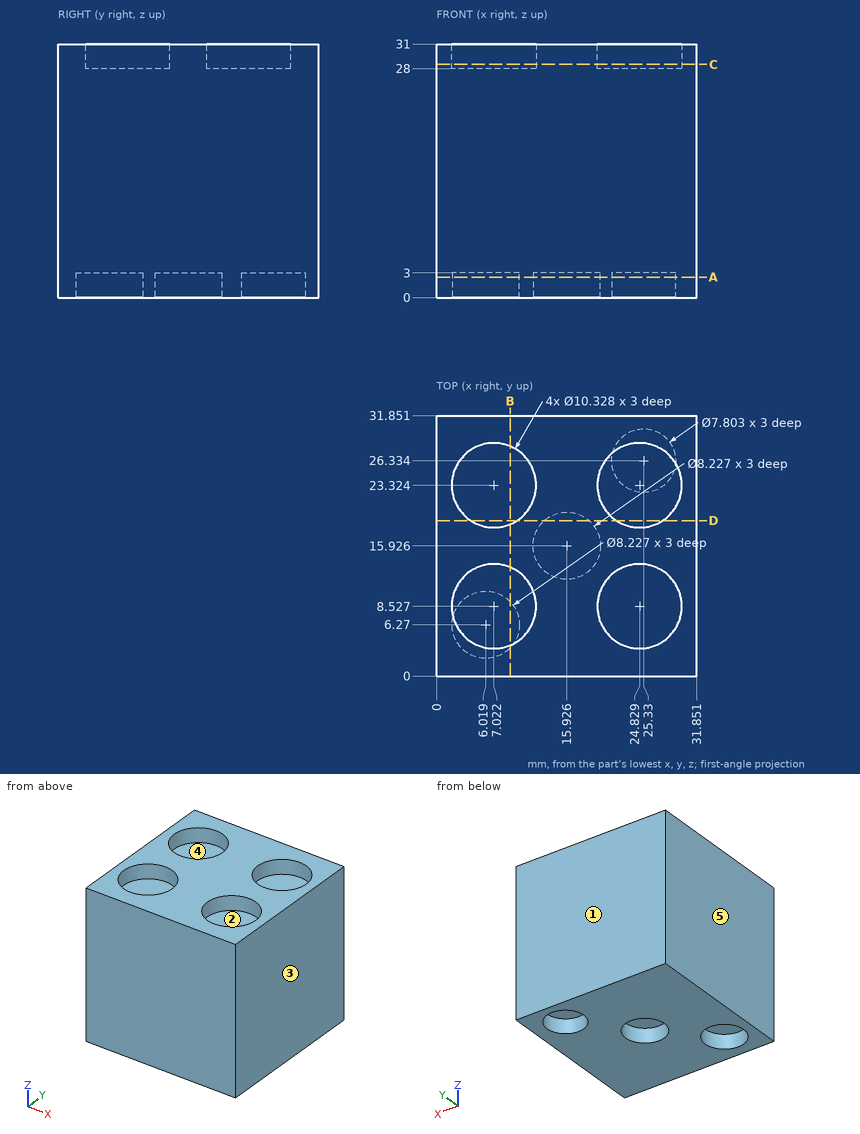
Verification items for this drawing (mm, ordinates from the low corner). A direction names the side the tool comes from. Round coordinates to 2 decimals unless told otherwise and drop trailing zeros. Order: outer loops, then holes, each group sorted by start corner. A loop starts at its lowest first (then second) coordinate and runs counter-clockwise, first axis right, second up. Notation, with made-up numbers: (2, 62.25) -> (50, 62.25) arc R16 ccw to (50, 88.25) -> close; hole circle Ø10 at (13, -34). An arc over 180 degrees is marked (long way). Use one line per item in the form item = value.
1. Mould release check, pull along Y, two halves, no side actions. Record for the marked faces 1, 2 and 3: pulls with the +Y half, pulls with the -Y half, needs draft (parallel to the pull), parting line crosses it, or undercut.
Working result:
face_1 = pulls with the +Y half
face_2 = undercut
face_3 = needs draft
2. Cross-section at C-C, the plane z = 28.5. Enter the section's corners in (x, y) (1 decimal).
Working result:
outline = (0, 0) -> (31.9, 0) -> (31.9, 31.9) -> (0, 31.9) -> close; hole circle Ø10.3 at (7, 8.5); hole circle Ø10.3 at (7, 23.3); hole circle Ø10.3 at (24.8, 8.5); hole circle Ø10.3 at (24.8, 23.3)
3. Set-up check for the marked faces 4 and 5: record each of +Z, -Z, +X, -X, +Y, -Y from which the full face is reachable in a straight line by a thin tool's end or side.
Working result:
face_4 = +Z
face_5 = +Z, -Z, -X, +Y, -Y
4. Cross-section at D-D, the plane y = 19. Enter the section's corners in (x, z) (1 decimal).
Working result:
outline = (0, 0) -> (13.2, 0) -> (13.2, 3) -> (18.7, 3) -> (18.7, 0) -> (31.9, 0) -> (31.9, 31) -> (27.7, 31) -> (27.7, 28) -> (22, 28) -> (22, 31) -> (9.8, 31) -> (9.8, 28) -> (4.2, 28) -> (4.2, 31) -> (0, 31) -> close
5. Cross-section at B-B, the plane x = 9. Enter the section's corners in (y, z) (1 decimal), plus the area to 3 significant figures.
Working result:
outline = (0, 0) -> (3.4, 0) -> (3.4, 3) -> (9.1, 3) -> (9.1, 0) -> (31.9, 0) -> (31.9, 31) -> (28.1, 31) -> (28.1, 28) -> (18.6, 28) -> (18.6, 31) -> (13.3, 31) -> (13.3, 28) -> (3.8, 28) -> (3.8, 31) -> (0, 31) -> close
area = 913 mm^2
6. Scan lines: line 1 along Z through (x, y) = (28.5, 27); line 2 along Z through (x, y) = (29, 23). Record each from-to range of solid material in increasing order. Write a range as from..to.
Working result:
line_1 = 3..31
line_2 = 0..28
7. Go/stop test with flat-tipped pins: pin 1 (16.5 mm diameter, centred on x = 7.02, y = 23.32, fed in from -Z); pin 2 (2.5 mm diameter, centred on x = 7, y = 5, fed in from -Z); pin 3 (5 mm diameter, centred on x = 7, y = 6.5, fed in from +Z). Record where each tip stops, or that it passes through.
Working result:
pin_1 = 0
pin_2 = 3
pin_3 = 28
8. Cross-section at A-A, the plane z = 2.5. Enter the section's corners in (x, y) (1 decimal).
Working result:
outline = (0, 0) -> (31.9, 0) -> (31.9, 31.9) -> (0, 31.9) -> close; hole circle Ø8.2 at (6, 6.3); hole circle Ø8.2 at (15.9, 15.9); hole circle Ø7.8 at (25.3, 26.3)
